Geometry: final body of the model. Coordinates: model frame, mm. Give positions to 0.01 mm unless a question says otherwise; leave off trailing zeros. Loops run counter-clockwise (first coordinate to the right, second up) from the corner with the lowest first, then second, coordinate; pieces in that order, holes last.
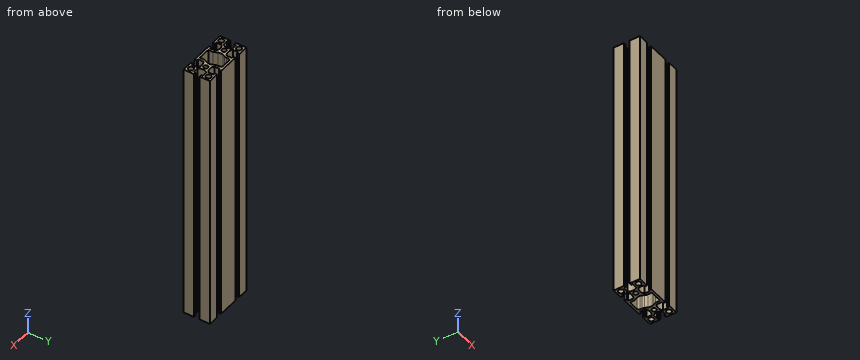
from build123d import *

# Parameters (mm, degrees)
F0_R     = 3
F0_R_2   = 2.5
F1_DEPTH = 295
F2_R     = 2
F3_R     = 7


# Not quite as in the source:
# - a feature names something its author has since deleted; it is built from what else it names


with BuildPart() as f1:
    # F0 (on Top) → F1 (new body)
    with BuildSketch(Plane.XY):
        with BuildLine():
            Line((18.15, -15), (30, -15))
            Line((30, -15), (30, -3.15))
            Line((30, -3.15), (27.5, -3.15))
            Line((27.5, -3.15), (27.5, -5.15))
            Line((27.5, -5.15), (21.5477069044, -5.15))
            ThreePointArc((21.5477069044, -5.15), (19.5, 0), (21.5477069044, 5.15))
            Line((21.5477069044, 5.15), (27.5, 5.15))
            Line((27.5, 5.15), (27.5, 3.15))
            Line((27.5, 3.15), (30, 3.15))
            Line((30, 3.15), (30, 15))
            Line((30, 15), (18.15, 15))
            Line((18.15, 15), (18.15, 12.5))
            Line((18.15, 12.5), (20.15, 12.5))
            Line((20.15, 12.5), (20.15, 6.5477069044))
            ThreePointArc((20.15, 6.5477069044), (15, 4.5), (9.85, 6.5477069044))
            Line((9.85, 6.5477069044), (9.85, 12.5))
            Line((9.85, 12.5), (11.85, 12.5))
            Line((11.85, 12.5), (11.85, 15))
            Line((11.85, 15), (-11.85, 15))
            Line((-11.85, 15), (-11.85, 12.5))
            Line((-11.85, 12.5), (-9.85, 12.5))
            Line((-9.85, 12.5), (-9.85, 6.5477069044))
            ThreePointArc((-9.85, 6.5477069044), (-15, 4.5), (-20.15, 6.5477069044))
            Line((-20.15, 6.5477069044), (-20.15, 12.5))
            Line((-20.15, 12.5), (-18.15, 12.5))
            Line((-18.15, 12.5), (-18.15, 15))
            Line((-18.15, 15), (-30, 15))
            Line((-30, 15), (-30, 3.15))
            Line((-30, 3.15), (-27.5, 3.15))
            Line((-27.5, 3.15), (-27.5, 5.15))
            Line((-27.5, 5.15), (-21.5477069044, 5.15))
            ThreePointArc((-21.5477069044, 5.15), (-19.5, 0), (-21.5477069044, -5.15))
            Line((-21.5477069044, -5.15), (-27.5, -5.15))
            Line((-27.5, -5.15), (-27.5, -3.15))
            Line((-27.5, -3.15), (-30, -3.15))
            Line((-30, -3.15), (-30, -15))
            Line((-30, -15), (-18.15, -15))
            Line((-18.15, -15), (-18.15, -12.5))
            Line((-18.15, -12.5), (-20.15, -12.5))
            Line((-20.15, -12.5), (-20.15, -6.5477069044))
            ThreePointArc((-20.15, -6.5477069044), (-15, -4.5), (-9.85, -6.5477069044))
            Line((-9.85, -6.5477069044), (-9.85, -12.5))
            Line((-9.85, -12.5), (-11.85, -12.5))
            Line((-11.85, -12.5), (-11.85, -15))
            Line((-11.85, -15), (11.85, -15))
            Line((11.85, -15), (11.85, -12.5))
            Line((11.85, -12.5), (9.85, -12.5))
            Line((9.85, -12.5), (9.85, -6.5477069044))
            ThreePointArc((9.85, -6.5477069044), (15, -4.5), (20.15, -6.5477069044))
            Line((20.15, -6.5477069044), (20.15, -12.5))
            Line((20.15, -12.5), (18.15, -12.5))
            Line((18.15, -12.5), (18.15, -15))
        make_face()
        with Locations((-25, -10)):
            Circle(F0_R, mode=Mode.SUBTRACT)
        with Locations((25, -10)):
            Circle(F0_R, mode=Mode.SUBTRACT)
        with Locations((-15, 0)):
            Circle(F0_R_2, mode=Mode.SUBTRACT)
        with Locations((-25, 10)):
            Circle(F0_R, mode=Mode.SUBTRACT)
        Polygon((-7, 7), (-7, 12.5), (0, 12.5), (7, 12.5), (7, 7), (10, 0), (7, -7), (7, -12.5), (0, -12.5), (-7, -12.5), (-7, -7), (-10, 0), align=None, mode=Mode.SUBTRACT)
        with Locations((15, 0)):
            Circle(F0_R_2, mode=Mode.SUBTRACT)
        with Locations((25, 10)):
            Circle(F0_R, mode=Mode.SUBTRACT)
    extrude(amount=F1_DEPTH)

    # F2
    f2_edges = [f1.edges().sort_by_distance(p)[0] for p in [
        (-7, 12.5, 147.5),
        (7, 12.5, 147.5),
    ]]
    fillet(f2_edges, radius=F2_R)

    # F3
    f3_edges = [f1.edges().sort_by_distance(p)[0] for p in [
        (-7, 7, 147.5),
        (-10, 0, 147.5),
        (7, 7, 147.5),
        (10, 0, 147.5),
    ]]
    fillet(f3_edges, radius=F3_R)


solid = f1.part
Item 1: Section query B-B on y = -10. Return loops of the section in (x, z), plus the area to 3 significant figures.
Values follow:
outline: (-30, 0) - (-28, 0) - (-28, 295) - (-30, 295) - close; (-22, 0) - (-20.15, 0) - (-20.15, 295) - (-22, 295) - close; (-9.85, 0) - (-7, 0) - (-7, 295) - (-9.85, 295) - close; (7, 0) - (9.85, 0) - (9.85, 295) - (7, 295) - close; (20.15, 0) - (22, 0) - (22, 295) - (20.15, 295) - close; (28, 0) - (30, 0) - (30, 295) - (28, 295) - close
area: 3,950 mm2
Item 2: Section query C-C on z = 213. Give the number of separate pieces and of enclosed holes in the cut face, plus the area to 3 significant figures.
Values follow:
separate pieces: 1
enclosed holes: 7
area: 710 mm2
Item 3: Ray query, probe 1 along X at (y, z) = (-13.25, 31.5); probe 2 along Y at (x, z) = (25, 105); probe 3 along Y at (x, z) = (15, 211). Return the intervals inside material, ascending.
Values follow:
probe 1: x = -30 to -18.15, -11.85 to 11.85, 18.15 to 30
probe 2: y = -15 to -13, -7 to -5.15, 5.15 to 7, 13 to 15
probe 3: y = -4.5 to -2.5, 2.5 to 4.5
Item 4: Pin query (flat end, axial travel): pin 1 (1.5 mm diameter, centred on y = -2, z = 54.5, fed in from -X). Return the tip coordinate at first contact, or that it passes through.
Values follow:
pin 1: stops at x = -20.02
Item 5: Section query A-A on x = 15. Return loops of the section in (y, z), plus the area to 3 significant figures.
Values follow:
outline: (-4.5, 0) - (-2.5, 0) - (-2.5, 295) - (-4.5, 295) - close; (2.5, 0) - (4.5, 0) - (4.5, 295) - (2.5, 295) - close
area: 1,180 mm2
